Job drawing, mm, ordinate dimensions from the low corner. One solid piece. Give positions to 0.01 mm unless a question says otherwise; leave off trailing zeros. Order: outer loops, then holes, each group sorted by start corner. A loop starts at its lowest first (then second) coordinate and runs counter-clockwise, first axis right, second up. Notation, with made-up numbers: M -12.5,-4.75 L 23.5,-4.75 A18 ccw 23.5,1.25 Z; hole C 30,0.5 d9. An arc over 180 degrees is marked long. One line per question, with ' | ' between items.
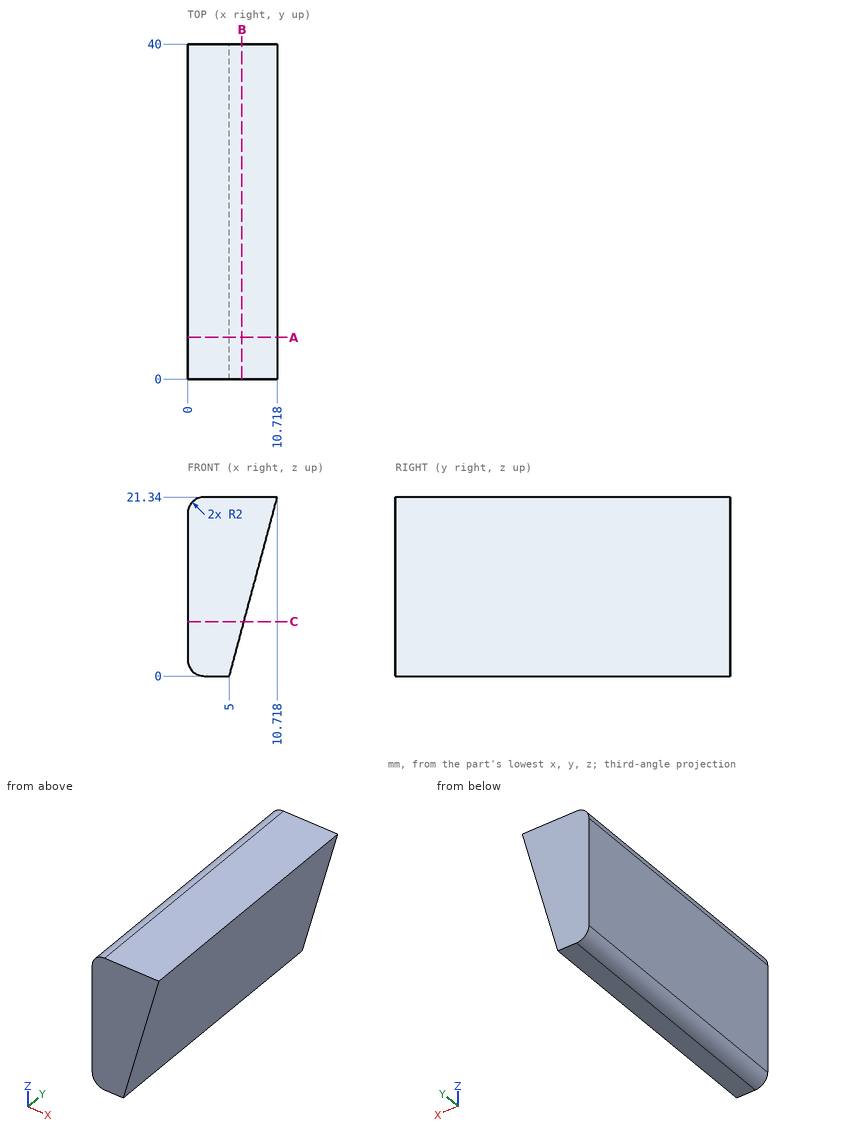
1. Slice it at C-C on z = 6.5. Give the cut face in (x, y).
Worked out:
outline: M 0,0 L 6.74,0 L 6.74,40 L 0,40 Z
2. Drop flat-ended pins along their axis: pin 1 (8 mm diameter, centred on y = 16, z = 16, fed in from +X); pin 2 (5 mm diameter, centred on y = 12.5, z = 10.5, fed in from +X); pin 3 (2 mm diameter, centred on y = 17, z = 13, fed in from +X). Give the stop position or say it passes through.
Worked out:
pin 1: stops at x = 10.36 | pin 2: stops at x = 8.48 | pin 3: stops at x = 8.75
3. Probe L1, parallel to X at y = 17, z = 9.75; L2, parallel to X at y = 12.5, z = 18.75. List the from-to ranges inside material, lowest first. Write a range as from..to.
Worked out:
L1: x = 0..7.61 | L2: x = 0..10.02
4. Slice it at B-B on x = 6.5. Give the cut face in (y, z).
Worked out:
outline: M 0,5.6 L 40,5.6 L 40,21.34 L 0,21.34 Z
5. Slice it at A-A on y = 5. Give the cut face in (x, z).
Worked out:
outline: M 0,2 A2 ccw 2,0 L 5,0 L 10.72,21.34 L 2,21.34 A2 ccw 0,19.34 Z
